Autodesk Inventor part; units mm, degrees
ref_plane "Work Plane1" through (0, 0, 0) normal (0, 0, 1) x (1, 0, 0)
ref_plane "YZ Plane" through (0, 0, 0) normal (1, 0, 0) x (0, 1, 0)
ref_plane "XZ Plane" through (0, 0, 0) normal (0, 1, 0) x (-1, 0, 0)
ref_plane "Work Plane1" through (0, 0, 0) normal (0, 0, 1) x (1, 0, 0)
sketch "Sketch1" plane through (0, 0, 0) normal (0, 0, 1) x (1, 0, 0)
  circle A0 centre (2.5, -19.5) radius 1
  circle A1 centre (2.5, -2.5) radius 1
  circle A2 centre (44.5, -2.5) radius 1
  circle A3 centre (44.5, -19.5) radius 1
  line L0 (0, -25) -> (0, 3)
  line L1 (0, -25) -> (47, -25)
  line L2 (47, -25) -> (47, 3)
  line L3 (0, 3) -> (47, 3)
  line L4 (5, 0) -> (42, 0)
  line L5 (42, 0) -> (42, -20)
  line L6 (42, -20) -> (5, -20)
  line L7 (5, -20) -> (5, 0)
  point P0 (0, 0)
extrude "Extrusion1" add sketch "Sketch1" along normal blind 3
sketch "Sketch2" plane through (0, 0, 3) normal (0, 0, 1) x (1, 0, 0)
  line L0 (47, 3) -> (0, 3)
  line L1 (47, 3) -> (0, 3)
  line L2 (0, 3) -> (0, 8)
  line L3 (0, 8) -> (47, 8)
  line L4 (47, 8) -> (47, 3)
  line L5 (0, -25) -> (47, -25)
  line L6 (0, -25) -> (47, -25)
  line L7 (47, -25) -> (47, -30)
  line L8 (47, -30) -> (0, -30)
  line L9 (0, -30) -> (0, -25)
  point P0 (0, 0)
  dimension "d2" = 5
  dimension "d3" = 5
extrude "Extrusion2" add sketch "Sketch2" against normal blind 3
sketch "Sketch4" plane through (0, 0, 3) normal (0, 0, 1) x (1, 0, 0)
  circle A0 centre (2.5, -2.5) radius 1
  circle A1 centre (44.5, -2.5) radius 1
  circle A2 centre (44.5, -19.5) radius 1
  circle A3 centre (2.5, -19.5) radius 1
  circle A4 centre (2.5, 5.5) radius 1
  circle A5 centre (44.5, 5.5) radius 1
  circle A6 centre (2.5, -27.5) radius 1
  circle A7 centre (44.5, -27.5) radius 1
  line L0 (0, 8) -> (47, 8)
  line L1 (47, -30) -> (0, -30)
  point P0 (0, 0)
  dimension "d6" = 2.5
  dimension "d7" = 2.5
  dimension "d8" = 2.5
  dimension "d9" = 2.5
extrude "Extrusion3" cut sketch "Sketch4" against normal blind 3 contours A4 | A5 | A6 | A7
properties part number "ProxSensor_Bracket_Back"
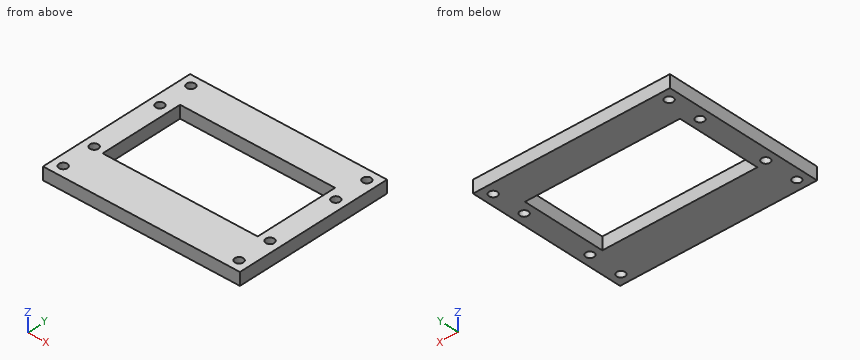
Could you check a few things on this model? Use its own coordinates, in mm. Give positions to 0.01 mm unless a question says otherwise; leave off trailing zeros. Order: outer loops, then holes, each group sorted by start corner. A loop starts at its lowest first (then second) coordinate and runs counter-clockwise, first axis right, second up.
1. Suppose I cut it at A-A (y = -14). List the corners of the cut face in (x, z) for me.
2. Suppose I cut it at B-B (z = 2.05). Give the number of separate pieces and of enclosed holes in the cut face, plus the area to 3 significant figures.
3. Suppose I cut it at C-C (x = 2.5). List the corners of the cut face in (y, z) for me.
4. Suppose I cut it at D-D (y = -19.5). List the corners of the cut face in (x, z) for me.
5. Will this pin go through, and if not, where does the flat tip stop? P1, Ø1.8, axis at x = 44.5, y = -27.5, coming from the +Z side.
6. I need wall thicknesses on L1, parallel to Y at x = 2.5, z = 1.75; L2, parallel to Y at x = 5.5, z = 1.9; L3, parallel to X at y = -7.5, z = 1.25. Which ranges of each line are inside material? Lowest first, please.
Solved:
1. outline: (0, 0) - (5, 0) - (5, 3) - (0, 3) - close; (42, 0) - (47, 0) - (47, 3) - (42, 3) - close
2. separate pieces: 1
2. enclosed holes: 9
2. area: 1,020 mm2
3. outline: (-30, 0) - (-28.5, 0) - (-28.5, 3) - (-30, 3) - close; (-26.5, 0) - (-20.5, 0) - (-20.5, 3) - (-26.5, 3) - close; (-18.5, 0) - (-3.5, 0) - (-3.5, 3) - (-18.5, 3) - close; (-1.5, 0) - (4.5, 0) - (4.5, 3) - (-1.5, 3) - close; (6.5, 0) - (8, 0) - (8, 3) - (6.5, 3) - close
4. outline: (0, 0) - (1.5, 0) - (1.5, 3) - (0, 3) - close; (3.5, 0) - (5, 0) - (5, 3) - (3.5, 3) - close; (42, 0) - (43.5, 0) - (43.5, 3) - (42, 3) - close; (45.5, 0) - (47, 0) - (47, 3) - (45.5, 3) - close
5. P1: passes through
6. L1: y = -30 to -28.5, -26.5 to -20.5, -18.5 to -3.5, -1.5 to 4.5, 6.5 to 8
6. L2: y = -30 to -20, 0 to 8
6. L3: x = 0 to 5, 42 to 47
